Check sheet for the modelled part. Datum: model origin and axes. Units: mm. Face numbers are marked on the shaded views. A direction names the side the tool comes from. Round coordinates to 2 decimals unless told otherwise and drop trailing zeros. Order: outer loops, then holes, each group sorted by start corner. A loop starts at its lowest first (then second) coordinate and runs counter-clockwise, first axis right, second up. Notation, with made-up numbers: (74.25, 32.5) -> (132.25, 32.5) arc R21 ccw to (132.25, 45.5) -> close; hole circle Ø2 at (53.5, -1.75). An arc over 180 degrees is marked (long way). Answer in a Markdown table with one row per item. Add a question column.
1. Material ranges on L1, parallel to Y at x = 0, z = 4.25; L2, parallel to X at y = -3.5, z = 6.5; L3, parallel to Z at x = -3.75, y = -1.5, recorded low to high. Write a range as from..to.
2. Sectioned sample at C-C, the plane x = -5. Record the boundary of the cut face in (y, z).
3. Access from +Z, -Z, +X, -X, +Y, -Y to the whole of each face (thin tool, end or side, straight path). Record for the marked faces 5, 6 and 7.
4. Sectioned sample at D-D, the plane y = -8.5. Record the boundary of the cut face in (x, z).
5. Draft check along Y on the marked faces 1, 2, 3 and 4. Enter one of: +Y half, -Y half, draft (parallel to the pull), parting line (faces both ways), or undercut.
6. Depth check by flat-ended pin: P1, Ø5.5, axis at x = -1.5, y = 4.5, coming from the +Z side; P2, Ø1.5, axis at x = 1, z = 17, coming from the -Y side; P3, Ø4.5, axis at x = 0, y = -3, coming from the -Z side; P4, Ø1.5, axis at x = -5, z = 33.5, coming from the +Y side. Enter the tip coordinate at first touch or a pass-through.
7. Sectioned sample at B-B, the plane y = 3.5. Record the boundary of the cut face in (x, z).
8. Sectioned sample at A-A, the plane z = 51. Record the boundary of the cut face in (x, y).
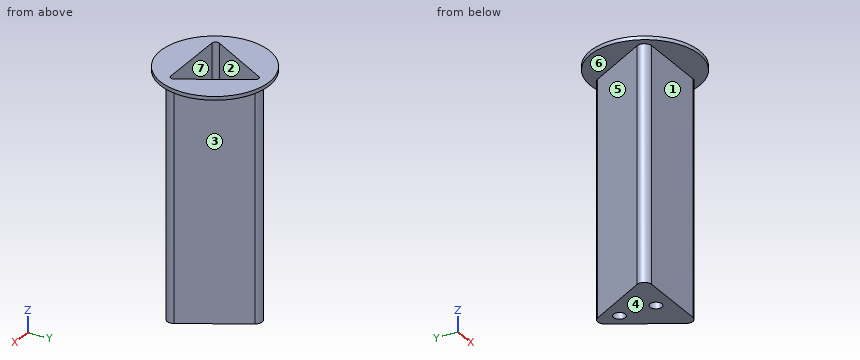
```python
from build123d import *

# Parameters (mm, degrees)
BOSS_EXTRUDE1_DEPTH       = 65
FILLET1_R                 = 2
M4X0_7_TAPPED_HOLE1_D     = 3.3
M4X0_7_TAPPED_HOLE1_DEPTH = 13
M4X0_7_TAPPED_HOLE1_TIP   = 0.991420021
SKETCH5_R                 = 15
BOSS_EXTRUDE3_DEPTH       = 1
SHELL2_START              = 1
SHELL2_OUTLINE_R          = 2.65
SHELL2_DEPTH              = 64
SHELL2_START_2            = 15.158053519
SHELL2_2_OUTLINE_R        = 2.65
SHELL2_2_DEPTH            = 49.841946481


with BuildPart() as part:
    # Sketch1 → Boss-Extrude1 (new body)
    with BuildSketch(Plane.XY):
        Polygon((-12.990381057, -7.5), (12.990381057, -7.5), (0, 15), align=None)
    extrude(amount=BOSS_EXTRUDE1_DEPTH)

    # Fillet1
    fillet1_edges = [part.edges().sort_by_distance(p)[0] for p in [
        (-12.990381057, -7.5, 32.5),
        (0, 15, 32.5),
        (12.990381057, -7.5, 32.5),
    ]]
    fillet(fillet1_edges, radius=FILLET1_R)

    # M4x0.7 Tapped Hole1
    with Locations(Plane(origin=(0, 0, 0), x_dir=(-1, 0, 0), z_dir=(0, 0, -1))):
        with Locations((0, -3), (0, 7)):
            Hole(M4X0_7_TAPPED_HOLE1_D / 2, depth=M4X0_7_TAPPED_HOLE1_DEPTH)
            with Locations((0, 0, -(M4X0_7_TAPPED_HOLE1_DEPTH + M4X0_7_TAPPED_HOLE1_TIP / 2))):  # 118° drill point
                Cone(0, M4X0_7_TAPPED_HOLE1_D / 2, M4X0_7_TAPPED_HOLE1_TIP, mode=Mode.SUBTRACT)

    # Sketch5 → Boss-Extrude3 (add)
    with BuildSketch(Plane.XY.offset(65)):
        Circle(SKETCH5_R)
    extrude(amount=-BOSS_EXTRUDE3_DEPTH)

    # Shell2: read off the stored shape, not the designer's step
    # Shell2 outline → Shell2 (cut)
    with BuildSketch(Plane.XY.offset(SHELL2_START)):
        with BuildLine():
            Line((-9.526279442, -6.5), (9.526279442, -6.5))
            ThreePointArc((9.526279442, -6.5), (10.392304845, -6), (10.392304845, -5))
            Line((10.392304845, -5), (0.866025404, 11.5))
            ThreePointArc((0.866025404, 11.5), (0, 12), (-0.866025404, 11.5))
            Line((-0.866025404, 11.5), (-10.392304845, -5))
            ThreePointArc((-10.392304845, -5), (-10.392304845, -6), (-9.526279442, -6.5))
        make_face()
        with Locations((0, -3)):
            Circle(SHELL2_OUTLINE_R, mode=Mode.SUBTRACT)
        with Locations((0, 7)):
            Circle(SHELL2_OUTLINE_R, mode=Mode.SUBTRACT)
    extrude(amount=SHELL2_DEPTH, mode=Mode.SUBTRACT)

    # Shell2 2 outline → Shell2 2 (cut)
    with BuildSketch(Plane.XY.offset(SHELL2_START_2)):
        with Locations((0, 7)):
            Circle(SHELL2_2_OUTLINE_R)
        with Locations((0, -3)):
            Circle(SHELL2_2_OUTLINE_R)
    extrude(amount=SHELL2_2_DEPTH, mode=Mode.SUBTRACT)

    # Shell2 3 outline → Shell2 3 (revolve, cut)
    with BuildSketch(Plane.XZ.offset(-7)):
        Polygon((2.65, 15.158053519), (0, 15.158053519), (2.65, 13.565772778), align=None)
    revolve(axis=Axis((0, 7, 0), (0, 0, 1)), mode=Mode.SUBTRACT)

    # Shell2 4 outline → Shell2 4 (revolve, cut)
    with BuildSketch(Plane.XZ.offset(3)):
        Polygon((2.65, 15.158053519), (0, 15.158053519), (2.65, 13.565772778), align=None)
    revolve(axis=Axis((0, -3, 0), (0, 0, 1)), mode=Mode.SUBTRACT)


solid = part.part
```
Answer key:
| question | item | result |
|---|---|---|
| 1 | L1 | y = -7.5..-6.5, -5.65..-4.65, -1.35..-0.35, 4.35..5.35, 8.65..9.65, 12..13 |
| 1 | L2 | x = -10.68..-9.53, -2.6..-1.57, 1.57..2.6, 9.53..10.68 |
| 1 | L3 | z = 0..1 |
| 2 | outline | (-14.14, 64) -> (-7.5, 64) -> (-7.5, 0) -> (6.34, 0) -> (6.34, 64) -> (14.14, 64) -> (14.14, 65) -> (4.34, 65) -> (4.34, 1) -> (-6.5, 1) -> (-6.5, 65) -> (-14.14, 65) -> close |
| 3 | face 5 | -Z, -X, +Y |
| 3 | face 6 | -Z |
| 3 | face 7 | +Z |
| 4 | outline | (-12.36, 64) -> (12.36, 64) -> (12.36, 65) -> (-12.36, 65) -> close |
| 5 | face 1 | -Y half |
| 5 | face 2 | undercut |
| 5 | face 3 | +Y half |
| 5 | face 4 | draft |
| 6 | P1 | stops at z = 15.06 |
| 6 | P2 | stops at y = -7.5 |
| 6 | P3 | stops at z = 0 |
| 6 | P4 | stops at y = 7.64 |
| 7 | outline | (-14.59, 64) -> (-6.64, 64) -> (-6.64, 0) -> (6.64, 0) -> (6.64, 64) -> (14.59, 64) -> (14.59, 65) -> (5.48, 65) -> (5.48, 1) -> (-5.48, 1) -> (-5.48, 65) -> (-14.59, 65) -> close |
| 8 | outline | (-11.26, -4.5) arc R2 ccw to (-9.53, -7.5) -> (9.53, -7.5) arc R2 ccw to (11.26, -4.5) -> (1.73, 12) arc R2 ccw to (-1.73, 12) -> close; hole (-10.39, -5) arc R1 ccw to (-9.53, -6.5) -> (9.53, -6.5) arc R1 ccw to (10.39, -5) -> (0.87, 11.5) arc R1 ccw to (-0.87, 11.5) -> close |
